The listing builds one solid part. Answer for the finished solid, in the listing's coordinates (mm). Face numbers are marked on the shaded views. A direction names the side the tool comes from. Coordinates: 2 decimals unless noted, no trailing zeros. Order: outer loops, then holes, each group sorted by start corner. A loop starts at its lowest first (then second) coordinate and runs counter-clockwise, first axis right, second up. Notation, with made-up numbers: (37.25, 60) -> (69.25, 60) arc R18 cw to (69.25, 88) -> close; hole circle Ø1 at (-20.75, 51.25). An arc over 180 degrees is marked (long way). Answer in a Markdown table with one row per item. Add a question column.
```python
from build123d import *

# Parameters (mm, degrees)
SKETCH1_R           = 2
SKETCH1_R_2         = 13.5
BOSS_EXTRUDE1_DEPTH = 2
SKETCH4_R           = 2
BOSS_EXTRUDE2_DEPTH = 4
CHAMFER1_SIZE       = 1.5
BOSS_EXTRUDE3_DEPTH = 2
FILLET2_R           = 0.75
FILLET4_R           = 0.75


with BuildPart() as part:
    # Sketch1 → Boss-Extrude1 (new body)
    with BuildSketch(Plane.XY):
        with BuildLine():
            Line((-15.5, -21), (15.5, -21))
            ThreePointArc((15.5, -21), (19.389087297, -19.389087297), (21, -15.5))
            Line((21, -15.5), (21, 15.5))
            ThreePointArc((21, 15.5), (19.389087297, 19.389087297), (15.5, 21))
            Line((15.5, 21), (-15.5, 21))
            ThreePointArc((-15.5, 21), (-19.389087297, 19.389087297), (-21, 15.5))
            Line((-21, 15.5), (-21, -15.5))
            ThreePointArc((-21, -15.5), (-19.389087297, -19.389087297), (-15.5, -21))
        make_face()
        with Locations((-15.5, 15.5)):
            Circle(SKETCH1_R, mode=Mode.SUBTRACT)
        with Locations(Location((-15.5, -15.5, 0), (0, 0, 180))):
            Circle(SKETCH1_R, mode=Mode.SUBTRACT)
        with Locations((15.5, -15.5)):
            Circle(SKETCH1_R, mode=Mode.SUBTRACT)
        with Locations(Location((15.5, 15.5, 0), (0, 0, 180))):
            Circle(SKETCH1_R, mode=Mode.SUBTRACT)
        Circle(SKETCH1_R_2, mode=Mode.SUBTRACT)
    extrude(amount=BOSS_EXTRUDE1_DEPTH)



with BuildPart() as body_2:
    # Sketch4 → Boss-Extrude2 (new body)
    with BuildSketch(Plane(origin=(0, -21, 0), x_dir=(1, 0, 0), z_dir=(0, 1, 0))):
        with BuildLine():
            Line((-15.5, 0), (-15.5, 5))
            ThreePointArc((-15.5, 5), (-17.110912703, 8.889087297), (-21, 10.5))
            Line((-21, 10.5), (-21, 31.5))
            ThreePointArc((-21, 31.5), (-17.110912703, 33.110912703), (-15.5, 37))
            Line((-15.5, 37), (-15.5, 42))
            Line((-15.5, 42), (15.5, 42))
            Line((15.5, 42), (15.5, 37))
            ThreePointArc((15.5, 37), (17.110912703, 33.110912703), (21, 31.5))
            Line((21, 31.5), (21, 10.5))
            ThreePointArc((21, 10.5), (17.110912703, 8.889087297), (15.5, 5))
            Line((15.5, 5), (15.5, 0))
            Line((15.5, 0), (15.5, -2))
            Line((15.5, -2), (-15.5, -2))
            Line((-15.5, -2), (-15.5, 0))
        make_face()
        with Locations(Location((-8, 31, 0), (0, 0, 270))):
            Circle(SKETCH4_R, mode=Mode.SUBTRACT)
        with Locations(Location((-8, 11, 0), (0, 0, 90))):
            Circle(SKETCH4_R, mode=Mode.SUBTRACT)
        with Locations(Location((8, 31, 0), (0, 0, 90))):
            Circle(SKETCH4_R, mode=Mode.SUBTRACT)
        with Locations(Location((8, 11, 0), (0, 0, 270))):
            Circle(SKETCH4_R, mode=Mode.SUBTRACT)
    extrude(amount=-BOSS_EXTRUDE2_DEPTH)

    # Chamfer1
    chamfer1_edges = [body_2.edges().sort_by_distance(p)[0] for p in [
        (-8, -21, -33),
        (-8, -21, -9),
        (8, -21, -29),
        (8, -21, -13),
    ]]
    chamfer(chamfer1_edges, length=CHAMFER1_SIZE)


with BuildPart() as part_1:
    add(part.part)

    add(body_2.part)  # Boss-Extrude3 merges body 2
    # Sketch5 → Boss-Extrude3 (add)
    with BuildSketch(Plane.ZY.offset(21)):
        Polygon((-26.5, -25), (2, 10.5), (2, 15.5), (-31.5, -25), align=None)
    boss_extrude3 = extrude(amount=BOSS_EXTRUDE3_DEPTH)

    # Mirror5: Boss-Extrude3 across plane
    add(boss_extrude3.mirror(Plane(origin=(0, 0, 0), x_dir=(0, 0, 1), z_dir=(1, 0, 0))))

    # Fillet2
    fillet2_edges = [part_1.edges().sort_by_distance(p)[0] for p in [
        (23, 13, 2),
    ]]
    fillet(fillet2_edges, radius=FILLET2_R)

    # Fillet4
    fillet4_edges = [part_1.edges().sort_by_distance(p)[0] for p in [
        (-23, 13, 2),
    ]]
    fillet(fillet4_edges, radius=FILLET4_R)


solid = part_1.part
```
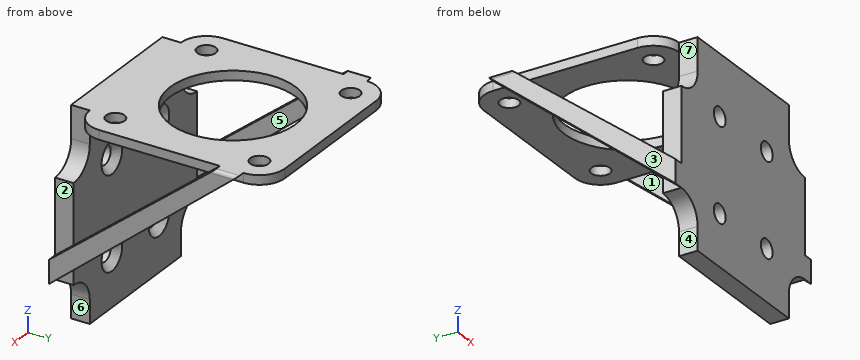
Q1. A cutting plane is placed at A-A (x = 0). Determine the outline of the cut face in (y, z).
Q2. A cutting plane is placed at B-B (y = 0). Determine the outline of the cut face in (x, z).
Q3. Straight lines are drawn through the part: line 1 (X direction, y = -23.9, z = -31); line 2 (X direction, y = -22, z = -32); line 3 (Y direction, x = 15, z = 1). For each, find the intervals that lie inside material, in ascending order.
Q4. A cutting plane is placed at C-C (y = -20). Determine the outline of the cut face in (x, z), then the cut area to 3 significant figures.
Q5. Determine the mould class of the marked faces 1, 2 and 3 for opening direction X: +X half, -X half, draft (parallel to the pull), parting line (faces both ways), or undercut.
Q6. Given pin 1 (4 mm diameter, centred on x = 3.5, y = 14.5, fed in from -Z); pin 2 (12 mm diameter, centred on x = -7, z = -27, fed in from +Y); pin 3 (1.6 mm diameter, centred on y = -4, z = 0.5, fed in from -X), each flat-ended and moving along its own axis, determine where each tip first touches the part or whether it passes through.
Q7. A cutting plane is placed at D-D (x = 8). Determine the outline of the cut face in (y, z), then the cut area to 3 significant figures.
Q8. For the marked faces 4, 5, 6 and 7, determine the directions among +Z, -Z, +X, -X, +Y, -Y from which every point of the face is accessible in a straight line to the end or side of a thin tool.
Returned:
| question | item | result |
|---|---|---|
| 1 | outline | (-25, -42) -> (-21, -42) -> (-21, 0) -> (-13.5, 0) -> (-13.5, 2) -> (-25, 2) -> close; (13.5, 0) -> (21, 0) -> (21, 2) -> (13.5, 2) -> close |
| 2 | outline | (-23, -10.82) -> (-21, -10.82) -> (-21, -6.43) -> (-23, -6.43) -> close; (-21, 0) -> (-13.5, 0) -> (-13.5, 2) -> (-21, 2) -> close; (13.5, 0) -> (21, 0) -> (21, 2) -> (13.5, 2) -> close; (21, -10.82) -> (23, -10.82) -> (23, -6.43) -> (21, -6.43) -> close |
| 3 | line 1 | x = -21 to -10, -6 to 6, 10 to 21 |
| 3 | line 2 | x = -18.71 to -10.29, -5.71 to 5.71, 10.29 to 18.71 |
| 3 | line 3 | y = -25 to -17.44, -13.56 to 13.56, 17.44 to 21 |
| 4 | outline | (-23, -27.36) -> (-21, -27.36) -> (-21, -22.49) -> (-23, -22.49) -> close; (-18.66, 0) -> (18.66, 0) -> (18.66, 2) -> (-18.66, 2) -> close; (21, -27.36) -> (23, -27.36) -> (23, -22.49) -> (21, -22.49) -> close |
| 4 | area | 94.2 mm² |
| 5 | face 1 | undercut |
| 5 | face 2 | +X half |
| 5 | face 3 | -X half |
| 6 | pin 1 | stops at z = 0 |
| 6 | pin 2 | stops at y = -21 |
| 6 | pin 3 | stops at x = -21 |
| 7 | outline | (-25, -42) -> (-21, -42) -> (-21, -34.5) -> (-22.5, -33) -> (-25, -33) -> close; (-25, -29) -> (-22.5, -29) -> (-21, -27.5) -> (-21, -14.5) -> (-22.5, -13) -> (-25, -13) -> close; (-25, -9) -> (-22.5, -9) -> (-21, -7.5) -> (-21, 0) -> (-10.87, 0) -> (-10.87, 2) -> (-25, 2) -> close; (10.87, 0) -> (21, 0) -> (21, 2) -> (10.87, 2) -> close |
| 7 | area | 180 mm² |
| 8 | face 4 | -Z, -X, +Y, -Y |
| 8 | face 5 | -Z, +Y |
| 8 | face 6 | -Z, +X, +Y, -Y |
| 8 | face 7 | +Z, -X, -Y |
